The listing builds one solid part. Answer for the finished solid, in the listing's coordinates (mm). Give positions to 0.01 mm unless a question says otherwise; leave off trailing zeros. Order: outer loops, then holes, each group sorted by start corner. A loop starts at its lowest first (then second) coordinate and runs counter-clockwise, first axis right, second up. Notation, with made-up numbers: (19.5, -32) -> (36.5, -32) arc R27 ccw to (36.5, -2) -> close; hole circle Ø6 at (59.5, 40.25). An arc over 180 degrees is marked (long way). Write item = value, one per line. Start each with the question number.
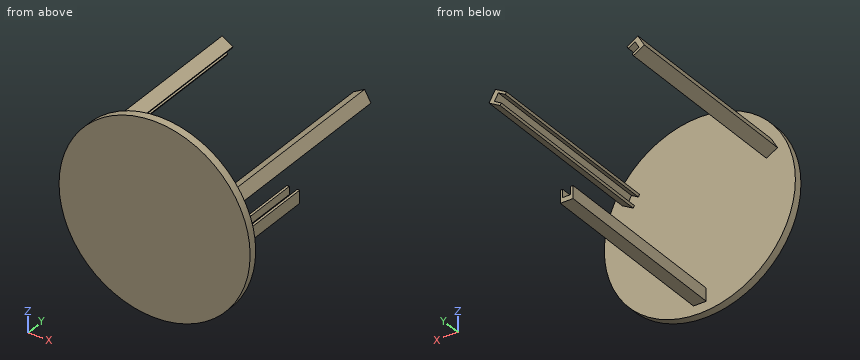
```python
from build123d import *

# Parameters (mm, degrees)
SKETCH2_R           = 300
BOSS_EXTRUDE1_DEPTH = 25
SKETCH4_W           = 40
SKETCH4_H           = 40
BOSS_EXTRUDE2_DEPTH = 600
SKETCH5_W           = 25
SKETCH5_H           = 25
CUT_EXTRUDE3_DEPTH  = 600
CIRPATTERN2_COUNT   = 3


with BuildPart() as part:
    # Sketch2 → Boss-Extrude1 (new body)
    with BuildSketch(Plane(origin=(0, 0, 0), x_dir=(1, 0, 0), z_dir=(0, 1, 0))):
        Circle(SKETCH2_R)
    extrude(amount=BOSS_EXTRUDE1_DEPTH)

    # Sketch4 → Boss-Extrude2 (add)
    with BuildSketch(Plane(origin=(0, 25, 0), x_dir=(1, 0, 0), z_dir=(0, 1, 0))):
        with Locations((0, 250)):
            Rectangle(SKETCH4_W, SKETCH4_H)
    boss_extrude2 = extrude(amount=BOSS_EXTRUDE2_DEPTH)

    # Sketch5 → Cut-Extrude3 (cut)
    with BuildSketch(Plane(origin=(0, 625, 0), x_dir=(1, 0, 0), z_dir=(0, 1, 0))):
        with Locations((-0.042882398, 242.5)):
            Rectangle(SKETCH5_W, SKETCH5_H)
    cut_extrude3 = extrude(amount=-CUT_EXTRUDE3_DEPTH, mode=Mode.SUBTRACT)

    # CirPattern2: Boss-Extrude2, Cut-Extrude3 ×3 about axis
    cirpattern2_axis = Axis((0, 0, 0), (0, 1, 0))
    for i in range(1, CIRPATTERN2_COUNT):
        add(boss_extrude2.rotate(cirpattern2_axis, i * 360 / CIRPATTERN2_COUNT))
        add(cut_extrude3.rotate(cirpattern2_axis, i * 360 / CIRPATTERN2_COUNT), mode=Mode.SUBTRACT)


solid = part.part
```
Item 1: Flat-ended cylindrical pins translate along their axes: pin 1 (20 mm diameter, centred on y = 228.5, z = -239.5, fed in from +X); pin 2 (12 mm diameter, centred on x = 224, z = -142, fed in from +Y); pin 3 (2.5 mm diameter, centred on x = 16.5, y = 254, fed in from +Z); pin 4 (10 mm diameter, centred on x = 27.5, y = 521.5, fed in from +Z). Find the tip coordinate at first contact, or state that the pin passes through.
Item 2: A cutting plane is placed at B-B, the plane x = 0. Write down the section's boundary in (y, z).
Item 3: Consider L1, parallel to Y at x = 225, z = -20.5; L2, parallel to Z at x = 16, y = 375.5; L3, parallel to X at y = 509, z = 134. Determine where each line is inside the solid, lowest interval first. Write a range as from..to.
Item 4: A cutting plane is placed at C-C, the plane z = 0. Write down the section's boundary in (x, y), plus the area to 3 significant figures.
Item 5: A cutting plane is placed at D-D, the plane x = 255.5. Write down the section's boundary in (y, z), plus the area to 3 significant figures.
Item 6: A cutting plane is placed at A-A, the plane y = 190. Write down the section's boundary in (x, z), plus the area to 4 significant figures.
Check values:
q1.pin_1 = 20
q1.pin_2 = 25
q1.pin_3 = -230
q1.pin_4 = through
q2.outline = (0, -300) -> (25, -300) -> (25, -270) -> (625, -270) -> (625, -255) -> (25, -255) -> (25, 300) -> (0, 300) -> close
q3.L1 = 0..25
q3.L2 = -270..-230
q3.L3 = -234.4..-217.08, -207.01..-192.09, 192.09..207.18, 217.08..234.4
q4.outline = (-300, 0) -> (300, 0) -> (300, 25) -> (-300, 25) -> close
q4.area = 15,000 mm^2
q5.outline = (0, -157.23) -> (25, -157.23) -> (25, 157.23) -> (0, 157.23) -> close
q5.area = 7,860 mm^2
q6.outline = (-243.83, 117.68) -> (-209.19, 97.68) -> (-205.41, 104.21) -> (-227.07, 116.71) -> (-214.57, 138.36) -> (-192.91, 125.86) -> (-189.19, 132.32) -> (-223.83, 152.32) -> close; (-20, -270) -> (20, -270) -> (20, -230) -> (12.46, -230) -> (12.46, -255) -> (-12.54, -255) -> (-12.54, -230) -> (-20, -230) -> close; (189.19, 132.32) -> (192.96, 125.79) -> (214.61, 138.29) -> (227.11, 116.64) -> (205.46, 104.14) -> (209.19, 97.68) -> (243.83, 117.68) -> (223.83, 152.32) -> close
q6.area = 2,925 mm^2
